Could you check a few things on this drawing? It's one solid part, dimensions in mm from its lowest x, y, z. Give positions to 0.01 mm unless a question says otherwise; leave off trailing zeros. Write each loop counter-clockwise with the first axis right and the second up, starting at its lowest first coordinate (ties: lowest second). Pieces come first, ordered by that corner, then holes. Notation, with made-up numbers: M 14.25,47 L 43.25,47 A17 ccw 43.25,72 Z; hole C 55.5,-38.75 d11. An arc over 180 degrees is marked long. Use CSV: the item, a comma, the result in double quotes. Start each with the question number.
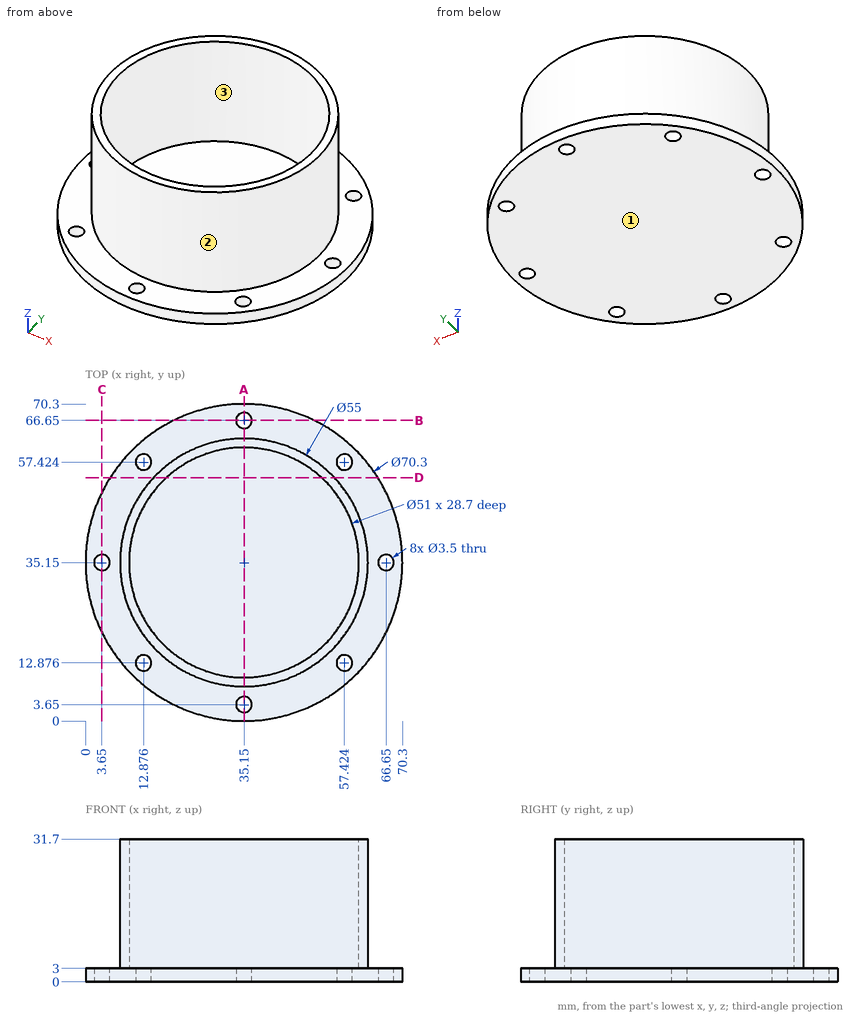
(1) Will these pins go through, and if not, where does the flat tip stop? pin 1 Ø15.5 at (x, y) = (40, 41) entering from +Z; pin 2 Ø6 at (y, z) = (13, 19) entering from +X; pin 3 Ø5 at (y, z) = (58.5, 4) entering from +X.
(2) Please list where these lines run through material, in increasing order: L1, parallel to Y at x = 35.15, z = 0.9; L2, parallel to X at y = 35, z = 14. Write a range as [from, to].
(3) I want a section at D-D (y = 54). Write out the boundary of the cut face in (x, z).
(4) I want a section at B-B (y = 66.65). Write out the boundary of the cut face in (x, z).
(5) I want a section at A-A (x = 35.15). Write out the boundary of the cut face in (y, z), and give its area (3 significant figures).
(6) Thinking about a two-plate mould opening in Y: for the marked faces 1, 2 and 3, which applies, released by +Y, released by -Y, zero draft, split by the parting line, or undercut?
Geometry results:
1,pin 1,"stops at z = 3"
1,pin 2,"stops at x = 54.89"
1,pin 3,"stops at x = 63.29"
2,L1,"y = [0, 1.9], [5.4, 64.9], [68.4, 70.3]"
2,L2,"x = [7.65, 9.65], [60.65, 62.65]"
3,outline,"M 5.48,0 L 64.82,0 L 64.82,3 L 55.17,3 L 55.17,31.7 L 52.32,31.7 L 52.32,3 L 17.98,3 L 17.98,31.7 L 15.13,31.7 L 15.13,3 L 5.48,3 Z"
4,outline,"M 19.55,0 L 33.4,0 L 33.4,3 L 19.55,3 Z; M 36.9,0 L 50.75,0 L 50.75,3 L 36.9,3 Z"
5,outline,"M 0,0 L 1.9,0 L 1.9,3 L 0,3 Z; M 5.4,0 L 64.9,0 L 64.9,3 L 62.65,3 L 62.65,31.7 L 60.65,31.7 L 60.65,3 L 9.65,3 L 9.65,31.7 L 7.65,31.7 L 7.65,3 L 5.4,3 Z; M 68.4,0 L 70.3,0 L 70.3,3 L 68.4,3 Z"
5,area,"305 mm2"
6,face 1,"zero draft"
6,face 2,"split by the parting line"
6,face 3,"undercut"
